Autodesk Inventor part; units mm, degrees
ref_plane "YZ Plane" through (0, 0, 0) normal (1, 0, 0) x (0, 1, 0)
ref_plane "XZ Plane" through (0, 0, 0) normal (0, 1, 0) x (-1, 0, 0)
ref_plane "XY Plane" through (0, 0, 0) normal (0, 0, 1) x (1, 0, 0)
sketch "Sketch1" plane through (0, 0, 0) normal (0, 0, 1) x (1, 0, 0)
  line L0 (-3.9, 0) -> (50.7, 0)
  line L1 (0, -3.9) -> (0, 50.7)
  line L2 (28.5, 0) -> (28.5, 27)
  line L3 (28.5, 27) -> (37, 27)
  line L4 (37, 27) -> (37, 36)
  line L5 (37, 36) -> (33.5, 36)
  line L6 (33.5, 36) -> (33.5, 33)
  line L7 (33.5, 33) -> (28.5, 33)
  line L8 (28.5, 33) -> (28.5, 39)
  line L9 (28.5, 39) -> (25.5, 39)
  line L10 (25.5, 39) -> (25.5, 29)
  line L11 (25.5, 29) -> (20, 29)
  line L12 (20, 29) -> (20, 26)
  line L13 (20, 26) -> (16, 26)
  line L14 (16, 26) -> (16, 23)
  line L15 (16, 23) -> (19, 21)
  line L16 (19, 21) -> (19, 2)
  line L17 (19, 2) -> (22, 0)
  line L18 (22, 0) -> (28.5, 0)
  dimension "d0" = 3
  dimension "d1" = 32
  dimension "d2" = 38
  dimension "d3" = 57
  dimension "d4" = 40
  dimension "d5" = 51
  dimension "d6" = 57
  dimension "d7" = 74
  dimension "d8" = 5
  dimension "d9" = 2
  dimension "d10" = 21
  dimension "d11" = 23
  dimension "d12" = 26
  dimension "d13" = 29
  dimension "d14" = 27
  dimension "d15" = 33
  dimension "d16" = 36
  dimension "d17" = 39
revolve "Revolution1" add sketch "Sketch1" angle 360 about axis through (0, -10, 0) along (0, 1, 0)
fillet "Fillet1" radius 2 1 edges at (-28.5, 27, 0)
sketch "Sketch2" plane through (0, 0, 0) normal (0, -1, 0) x (1, 0, 0)
  circle A0 centre (0, 0) radius 28.5
  line L0 (-44.4, 0) -> (59.2, 0)
  line L1 (0, -44.4) -> (0, 59.2)
  line L2 (0, 32.909) -> (28.5, 16.4545)
  line L3 (28.5, 16.4545) -> (28.5, -16.4545)
  line L4 (28.5, -16.4545) -> (0, -32.909)
  line L5 (0, -32.909) -> (-28.5, -16.4545)
  line L6 (-28.5, -16.4545) -> (-28.5, 16.4545)
  line L7 (-28.5, 16.4545) -> (0, 32.909)
extrude "Extrusion1" add sketch "Sketch2" against normal blind 17 contours L3 L4 A0 | A0 L2 L3 | A0 L1 L2 | L4 L1 A0 | A0 L7 L1 | L1 L5 A0 | L6 L7 A0 | A0 L5 L6
thread "Thread1"
sketch "Sketch3" plane through (0, 36, 0) normal (0, 1, 0) x (1, 0, 0)
  circle A0 centre (0, 0) radius 37
  line L0 (-59.2, 0) -> (44.4, 0)
  line L1 (0, 44.4) -> (0, -59.2)
  line L2 (35.8887, 9) -> (39, 9)
  arc A1 (39, -9) -> (39, 9) centre (39, 0) ccw
  line L3 (39, -9) -> (35.8887, -9)
  dimension "d24" = 9
  dimension "d25" = 78
extrude "Extrusion2" add sketch "Sketch3" against normal blind 9 contours A0 L2 A1 L3
fillet "Fillet2" radius 2 2 edges at (35.8887, 31.5, 9) (35.8887, 31.5, -9)
sketch "Sketch4" plane through (39, 36, 0) normal (0, 1, 0) x (1, 0, 0)
  arc A0 (0, -9) -> (0, 9) centre (0, 0) ccw
hole "Hole1" at (39, 36, 0) direction (0, -1, 0) diameter 9 end through all
pattern_circular "Circular Pattern1" count 6 over 360 about axis through (0, 11.5, 0) along (0, -1, 0) of "Extrusion2", "Fillet2", "Hole1"
properties part number "Body Cap" material "Bronze, Soft Tin"
For this review, take the finished solid that the model builds, in its own axes (mm). A direction names the side the tool comes from. Coordinates: 2 decimals unless noted, no trailing zeros. Write each loop counter-clockwise with the first axis right and the second up, starting at its lowest first coordinate (ties: lowest second). Pieces come first, ordered by that corner, then holes.
(1) For pin 1 Ø12 at (y, z) = (7, -7) entering from +X; pin 2 Ø15.5 at (x, z) = (-10, -9) entering from +Y; pin 3 Ø1.3 at (x, y) = (-38, 32.5) entering from -Z; pin 4 Ø20 at (x, z) = (4.5, -3.5) entering from +Y, all flat-tipped, find the tip position at first contact; note any pin that passes through.
(2) The part is to be moulded in two halves that separate along Y. For faces 5 (the face through (-8.98, 26, -13.43)), 6 (the face through (-5.5, 33.9, -24.9)), 7 (the face through (-26, 17, 14)), say which applies: +Y half, -Y half, draft (parallel to the pull), parting line (faces both ways), or undercut.
(3) Add section A-A on y = 14. Give the boundary of the cut face in (x, z), then the cut area to 3 significant figures.
(4) Tool access review of faces 1 (the face through (-28.5, 8, 0)), 2 (the face through (-14.449, 8.381, 24.567)), 3 (the face through (10, 33, -27)), 4 (the face through (26, 17, -15)): name each direction out of +Z, -Z, +X, -X, +Y, -Y from which nothing blocks a thin tool from reaching the whole face with its end or side.
(5) Wall thickness on probe 1 along X at (y, z) = (27.6, 0); probe 2 along Z at (x, y) = (0, 34); probe 3 along X at (y, z) = (35, 0): over which ranges is each line inside the solid? List them lowest first.
Answer sheet:
1. pin 1: stops at x = 28.5
1. pin 2: stops at y = 29
1. pin 3: stops at z = -9
1. pin 4: passes through
2. face 5: +Y half
2. face 6: draft
2. face 7: undercut
3. outline: (-28.5, -16.45) - (0, -32.91) - (28.5, -16.45) - (28.5, 16.45) - (0, 32.91) - (-28.5, 16.45) - close; hole circle Ø38 at (0, 0)
3. area: 1,680 mm2
4. face 1: +Z, -Z, -X, -Y
4. face 2: +Z, -X, -Y
4. face 3: +Y
4. face 4: -Z, +X
5. probe 1: x = -48 to -43.5, -34.5 to -20, 20 to 34.5, 43.5 to 48
5. probe 2: z = -37 to -33.5, -28.5 to -25.5, 25.5 to 28.5, 33.5 to 37
5. probe 3: x = -48 to -43.5, -34.5 to -33.5, -28.5 to -25.5, 25.5 to 28.5, 33.5 to 34.5, 43.5 to 48
